Design review of the part built by this model. Coordinates are the model's own, in mm. A direction names the side the tool comes from. Coordinates: 2 decimals unless noted, no trailing zeros. Order: outer loops, then holes, each group sorted by start corner. A loop starts at its lowest first (then second) coordinate and runs counter-clockwise, first axis right, second up. Notation, with made-up numbers: M -25.75,13 L 17.25,13 A30 cw 17.25,38 Z; hole C 60.5,52.5 d10. An arc over 180 degrees is marked long. Answer in a Markdown table with one row per item.
Autodesk Inventor part; units mm, degrees
ref_plane "Work Plane1" through (-15.24, 0, -101.6) normal (-1, 0, 0) x (0, 0, 1)
ref_plane "YZ Plane" through (0, 0, 0) normal (1, 0, 0) x (0, 1, 0)
ref_plane "XZ Plane" through (0, 0, 0) normal (0, 1, 0) x (-1, 0, 0)
sketch "Sketch1" plane through (0, 0, 0) normal (0, 1, 0) x (-1, 0, 0)
  line L0 (0, 0) -> (30.48, 0)
  line L1 (30.48, 0) -> (30.48, -101.6)
  line L2 (30.48, -101.6) -> (0, -101.6)
  line L3 (0, -101.6) -> (0, 0)
  circle A0 centre (15.24, -16.51) radius 4.1275
  circle A1 centre (15.24, -85.09) radius 4.1275
  dimension "d0" = 30.48
  dimension "d1" = 101.6
  dimension "d4" = 8.255
  dimension "d5" = 8.255
extrude "Extrusion1" add sketch "Sketch1" along normal blind 7.62
sketch "Sketch2" plane through (0, 0, 0) normal (1, 0, 0) x (0, 0, -1)
  line L0 (0, 0) -> (0, 7.62)
  line L1 (0, 7.62) -> (101.6, 7.62)
  line L2 (0, 7.62) -> (101.6, 7.62)
  arc A0 (51.8409, 19.4967) -> (49.7591, 19.4967) centre (50.8, 25.4) ccw
  arc A1 (44.3162, 18.9162) -> (57.2837, 18.9163) centre (50.8, 25.4) ccw
  line L3 (50.8, 25.4) -> (59.9694, 25.4) construction
  line L4 (50.8, 25.4) -> (59.9694, 25.4) construction
  arc A2 (45.4388, 20.0388) -> (44.3162, 18.9162) centre (44.8775, 19.4775) ccw
  arc A3 (57.2837, 18.9163) -> (56.1612, 20.0388) centre (56.7225, 19.4775) ccw
  line L5 (50.8, 25.4) -> (58.3819, 25.4) construction
  arc A4 (48.1597, 18.2927) -> (49.7591, 19.4967) centre (48.3236, 19.7391) ccw
  arc A5 (51.8409, 19.4967) -> (53.4403, 18.2927) centre (53.2763, 19.7391) ccw
  arc A6 (45.4388, 20.0388) -> (48.1597, 18.2927) centre (50.8, 25.4) ccw
  arc A7 (53.4403, 18.2927) -> (56.1612, 20.0388) centre (50.8, 25.4) ccw
  line L6 (50.8, 7.62) -> (22.225, 7.62)
  arc A8 (54.8949, 38.7005) -> (46.7051, 38.7005) centre (50.8, 36.195) ccw
  line L7 (22.225, 7.62) -> (46.7051, 38.7005)
  line L8 (50.8, 7.62) -> (79.375, 7.62)
  line L9 (79.375, 7.62) -> (54.8949, 38.7005)
  dimension "d16" = 28.575
  dimension "d17" = 28.575
extrude "Extrusion2" add sketch "Sketch2" against normal blind 6.35
ref_plane "Work Plane1" through (-15.24, 0, -101.6) normal (-1, 0, 0) x (0, 0, 1)
mirror "Mirror1" about plane through (-15.24, 0, -101.6) normal (-1, 0, 0) of "Extrusion2"
fillet "Fillet1" radius 12.7 4 edges at (-3.175, 7.62, -79.375) (-27.305, 7.62, -79.375) (-27.305, 7.62, -22.225) (-3.175, 7.62, -22.225)
fillet "Fillet3" radius 3.175 2 edges at (-24.13, 7.62, -50.8) (-6.35, 7.62, -50.8)
properties part number "TestingBracket"
(1) For faces 1 (the cylindrical face through (-23.22, 8.57, -50.31)), 2 (the cylindrical face through (-3.13, 16.23, -50.7)), 3 (the flat face through (-27.349, 25.765, -65.083)), 4 (the flat face through (-15, 7.62, -50)), list the 3-axis set-ups (+Z, -Z, +X, -X, +Y, -Y) from which the entire face can be reached by the end or side of a thin tool; tool diameter is ignored.
Return value:
| item | result |
|---|---|
| face 1 | +Z, -Z, +Y |
| face 2 | +X, -X |
| face 3 | -Z, +X, -X, +Y |
| face 4 | +Y |
(2) Add section D-D, the plane x = -5. Give the boundary of the cut face in (y, z) (1 decimal).
Return value:
| item | result |
|---|---|
| outline | M 0,-101.6 L 7.6,-101.6 L 7.6,-85.5 A12.7 cw 12.5,-75.6 L 38.7,-54.9 A4.8 ccw 38.7,-46.7 L 12.5,-26 A12.7 cw 7.6,-16.1 L 7.6,0 L 0,0 Z; hole M 18.3,-53.4 A1.5 cw 19.5,-51.8 A6 ccw long 19.5,-49.8 A1.5 cw 18.3,-48.2 A7.6 cw 20,-45.4 A0.8 ccw 18.9,-44.3 A9.2 ccw 18.9,-57.3 A0.8 ccw 20,-56.2 A7.6 cw Z |
(3) Add section B-B, the plane z = -50.8. Give the boundary of the cut face in (x, y) (3 decimals), and give its area (3 significant figures).
Return value:
| item | result |
|---|---|
| outline | M -30.48,0 L 0,0 L 0,16.231 L -6.35,16.231 L -6.35,10.795 A3.175 cw -9.525,7.62 L -20.955,7.62 A3.175 cw -24.13,10.795 L -24.13,16.231 L -30.48,16.231 Z; M -30.48,31.394 L -24.13,31.394 L -24.13,40.996 L -30.48,40.996 Z; M -6.35,31.394 L 0,31.394 L 0,40.996 L -6.35,40.996 Z |
| area | 468 mm2 |
(4) Insertion check: pin 1 Ø4 at (x, y) = (-5, 11.5) entering from -Z; pin 2 Ø8 at (x, z) = (-24.5, -87.5) entering from +Y. Each pin has a flat end and moves straight along its axis. Give the tip position at first contact, or say it passes through.
Return value:
| item | result |
|---|---|
| pin 1 | stops at z = -78.89 |
| pin 2 | stops at y = 7.78 |
(5) Draft analysis for pull direction Z (two halves, no side actions). For faces 5 (the cylindrical face through (-3.77, 8.93, -21.68)), 6 (the cylindrical face through (-27.35, 16.23, -50.9)), 7 (the cylindrical face through (-3.771, 8.86, -80.066)), state which applies: pulls with the +Z half, pulls with the -Z half, needs draft (parallel to the pull), parting line crosses it, or undercut.
Return value:
| item | result |
|---|---|
| face 5 | pulls with the +Z half |
| face 6 | undercut |
| face 7 | pulls with the -Z half |
(6) For line 1 along Z through (x, y) = (-15, 2); line 2 along Y through (x, z) = (-28.25, -50.8); line 3 along X through (y, z) = (18, -35.5), list the stretches that pass through material, from the lowest coordinate up. Write a range as from..to.
Return value:
| item | result |
|---|---|
| line 1 | z = -101.6..-89.21, -80.97..-20.63, -12.39..0 |
| line 2 | y = 0..16.23, 31.39..41 |
| line 3 | x = -30.48..-24.13, -6.35..0 |
(7) Add section C-C, the plane y = 36.5. Give the boundary of the cut face in (x, z).
Return value:
| item | result |
|---|---|
| outline | M -30.48,-56.63 L -24.13,-56.63 L -24.13,-44.97 L -30.48,-44.97 Z; M -6.35,-56.63 L 0,-56.63 L 0,-44.97 L -6.35,-44.97 Z |
(8) Add section A-A, the plane x = -15.24. Give the boundary of the cut face in (y, z), and give its area (3 significant figures).
Return value:
| item | result |
|---|---|
| outline | M 0,-101.6 L 7.62,-101.6 L 7.62,-89.22 L 0,-89.22 Z; M 0,-80.96 L 7.62,-80.96 L 7.62,-20.64 L 0,-20.64 Z; M 0,-12.38 L 7.62,-12.38 L 7.62,0 L 0,0 Z |
| area | 648 mm2 |
